Work out the finished part from the listing and answer in its coordinate system (mm). A direction names the side the tool comes from. Give positions to 0.01 mm unless a question says otherwise; leave off trailing zeros. Order: outer loops, then holes, each group sorted by start corner. A loop starts at its lowest first (then second) coordinate and runs counter-clockwise, first axis right, second up.
```python
from build123d import *

# Parameters (mm, degrees)
F0_W        = 65
F0_H        = 56
F1_DEPTH    = 41
F2_T        = -3
F3_W        = 5.12
F3_H        = 12.5
F4_DEPTH    = 4.318
F5_W        = 3.9
F5_H        = 31
F6_DEPTH    = 2
F7_W        = 3.9
F7_H        = 31
F8_DEPTH    = 2
F9_T1_DEPTH = 47.7630546142
F11_DEPTH   = 66.294
F12_W       = 8
F12_H       = 50
F13_DEPTH   = 14.732
F14_W       = 8.89
F14_H       = 2.41
F14_W_2     = 7.2
F15_DEPTH   = 25
F16_W       = 7.2
F16_H       = 2.41
F17_DEPTH   = 0.8
F18_W       = 32.2036024
F18_H       = 3
F19_DEPTH   = 25
F20_W       = 32.2036024
F20_H       = 3
F21_DEPTH   = 3.5
F22_W       = 65
F22_H       = 1.6
F23_DEPTH   = 1
F23_TAPER   = -30
F25_DEPTH   = 0.8
F26_W       = 8.89
F26_H       = 2.41
F27_DEPTH   = 0.8
F28_W       = 0.5773502692
F28_H       = 2.7547005384
F29_DEPTH   = 25
F30_W       = 3
F30_H       = 27.2
F30_H_2     = 28.8
F31_DEPTH   = 6


# Not quite as in the source:
# - a fillet or chamfer that OpenCascade refuses, or shapes differently, is made with other operations: its cross-section is extruded or revolved along the edge and cut away or added


with BuildPart() as f1:
    # F0 (on Top) → F1 (new body)
    with BuildSketch(Plane.XY):
        with Locations((-1.2741552845, -5.3390697837)):
            Rectangle(F0_W, F0_H)
    extrude(amount=F1_DEPTH)

    # F2
    f2_openings = [f1.faces().sort_by_distance(p)[0] for p in [
        (31.225845, -5.33907, 20.5),
    ]]
    offset(amount=F2_T, openings=f2_openings)

    # F3 (on face) → F4 (cut)
    with BuildSketch(Plane(origin=(-33.7741552845, 0, 0), x_dir=(0, -1, 0), z_dir=(-1, 0, 0))):
        with Locations((-7.7209302163, 19.25)):
            Rectangle(F3_W, F3_H)
        with Locations((11.3990697837, 19.25)):
            Rectangle(F3_W, F3_H)
    extrude(amount=-F4_DEPTH, mode=Mode.SUBTRACT)

    # F5 (on face) → F6 (join)
    with BuildSketch(Plane(origin=(0, 22.6609302163, 0), x_dir=(-1, 0, 0), z_dir=(0, 1, 0))):
        with Locations((-24.2758447155, 20.5)):
            Rectangle(F5_W, F5_H)
    extrude(amount=F6_DEPTH)

    # F7 (on face) → F8 (join)
    with BuildSketch(Plane.XZ.offset(33.3390697837)):
        with Locations((24.2758447155, 20.5)):
            Rectangle(F7_W, F7_H)
    extrude(amount=F8_DEPTH)

    # F9: fillet of radius 3.81 on 2 edges, made by hand

    # F9_s2 → F9_t1 (cut)
    with BuildSketch(Plane.XY.offset(-3.3815273071)):
        with BuildLine():
            ThreePointArc((22.3258447155, 22.6609302163), (23.7265335088, 24.1229479424), (25.6784556384, 24.6609302163))
            Line((25.6784556384, 24.6609302163), (22.3258447155, 24.6609302163))
            Line((22.3258447155, 24.6609302163), (22.3258447155, 22.6609302163))
        make_face()
        with BuildLine():
            ThreePointArc((22.3258447155, -33.3390697837), (23.7265335088, -34.8010875098), (25.6784556384, -35.3390697837))
            Line((25.6784556384, -35.3390697837), (22.3258447155, -35.3390697837))
            Line((22.3258447155, -35.3390697837), (22.3258447155, -33.3390697837))
        make_face()
    extrude(amount=F9_T1_DEPTH, mode=Mode.SUBTRACT)

    # F10 (on face) → F11 (cut)
    with BuildSketch(Plane(origin=(0, 22.6609302163, 0), x_dir=(-1, 0, 0), z_dir=(0, 1, 0))):
        Polygon((0.9777576845, 38), (-31.2258447155, 38), (-31.2258447155, 3), (0.9777576845, 3), (0.9777576845, 4), (-28.0222423155, 4), (-28.0222423155, 37), (0.9777576845, 37), align=None)
    extrude(amount=-F11_DEPTH, mode=Mode.SUBTRACT)

    # F12 (on face) → F13 (cut)
    with BuildSketch(Plane.XY.offset(41)):
        with Locations((27.2258447155, -5.3390697837)):
            Rectangle(F12_W, F12_H)
    extrude(amount=-F13_DEPTH, mode=Mode.SUBTRACT)

    # F14 (on face) → F15 (cut)
    with BuildSketch(Plane.XY.offset(41)):
        with Locations((-1.8741552845, 1.0109302163)):
            Rectangle(F14_W, F14_H)
        with BuildLine():
            ThreePointArc((-13.7741552845, -8.0290697837), (-11.8720380431, -7.2411870251), (-11.0841552845, -5.3390697837))
            ThreePointArc((-11.0841552845, -5.3390697837), (-11.8720380431, -3.4369525423), (-13.7741552845, -2.6490697837))
            ThreePointArc((-13.7741552845, -2.6490697837), (-15.6762725259, -3.4369525423), (-16.4641552845, -5.3390697837))
            ThreePointArc((-16.4641552845, -5.3390697837), (-15.6762725259, -7.2411870251), (-13.7741552845, -8.0290697837))
        make_face()
        with Locations((-1.8741552845, -11.6890697837)):
            Rectangle(F14_W_2, F14_H)
        with BuildLine():
            ThreePointArc((-16.4641552845, -5.3390697837), (-15.6762725259, -3.4369525423), (-13.7741552845, -2.6490697837))
            Line((-13.7741552845, -2.6490697837), (-16.4641552845, -2.6490697837))
            Line((-16.4641552845, -2.6490697837), (-16.4641552845, -5.3390697837))
        make_face()
        with BuildLine():
            Line((-16.4641552845, -8.0290697837), (-13.7741552845, -8.0290697837))
            ThreePointArc((-13.7741552845, -8.0290697837), (-15.6762725259, -7.2411870251), (-16.4641552845, -5.3390697837))
            Line((-16.4641552845, -5.3390697837), (-16.4641552845, -8.0290697837))
        make_face()
    extrude(amount=-F15_DEPTH, mode=Mode.SUBTRACT)

    # F16 (on face) → F17 (cut)
    with BuildSketch(Plane(origin=(0, 0, 38), x_dir=(1, 0, 0), z_dir=(0, 0, -1))):
        Polygon((-30.7741552845, 12.0888292812), (-30.7741552845, 11.2888292812), (-8.9876995774, 11.2888292812), (-5.4741552845, 10.0590887787), (1.7258447155, 10.0590887787), (5.2393890084, 11.2888292812), (23.2258447155, 11.2888292812), (23.2258447155, 12.0888292812), (5.2393890084, 12.0888292812), (1.7258447155, 13.3185697837), (-5.4741552845, 13.3185697837), (-8.9876995774, 12.0888292812), align=None)
        with Locations((-1.8741552845, 11.6890697837)):
            Rectangle(F16_W, F16_H, mode=Mode.SUBTRACT)
    extrude(amount=-F17_DEPTH, mode=Mode.SUBTRACT)

    # F18 (on face) → F19 (cut)
    with BuildSketch(Plane(origin=(0, 0, 38), x_dir=(1, 0, 0), z_dir=(0, 0, -1))):
        with Locations((15.1240435155, -21.1609302163)):
            Rectangle(F18_W, F18_H)
        Polygon((-0.9777576845, 33.3390697837), (-0.9777576845, 30.3390697837), (23.2258447155, 30.3390697837), (31.2258447155, 30.3390697837), (31.2258447155, 33.3390697837), align=None)
    extrude(amount=-F19_DEPTH, mode=Mode.SUBTRACT)

    # F20 (on face) → F21 (cut)
    with BuildSketch(Plane(origin=(0, 0, 0), x_dir=(1, 0, 0), z_dir=(0, 0, -1))):
        with Locations((15.1240435155, -21.1609302163)):
            Rectangle(F20_W, F20_H)
        with Locations((15.1240435155, 31.8390697837)):
            Rectangle(F20_W, F20_H)
    extrude(amount=-F21_DEPTH, mode=Mode.SUBTRACT)

    # F22 (on face) → F23 (join)
    with BuildSketch(Plane(origin=(0, 0, 0), x_dir=(1, 0, 0), z_dir=(0, 0, -1))):
        with Locations((-1.2741552845, 5.3390697837)):
            Rectangle(F22_W, F22_H)
    extrude(amount=F23_DEPTH, taper=F23_TAPER)

    # F24 (on face) → F25 (cut)
    with BuildSketch(Plane(origin=(0, 0, 38), x_dir=(1, 0, 0), z_dir=(0, 0, -1))):
        Polygon((23.2258447155, 3.6890697837), (23.2258447155, 6.9890697837), (-8.1741552845, 6.9890697837), (-8.9247106344, 8.2890697837), (-8.9247106344, 8.7890697837), (-19.4271999345, 8.7890697837), (-19.4271999345, 1.8890697837), (-8.9247106344, 1.8890697837), (-8.9247106344, 2.3890697837), (-8.1741552845, 3.6890697837), align=None)
        with BuildLine():
            Line((-16.4641552845, 8.0290697837), (-13.7741552845, 8.0290697837))
            ThreePointArc((-13.7741552845, 8.0290697837), (-11.0841552845, 5.3390697837), (-13.7741552845, 2.6490697837))
            Line((-13.7741552845, 2.6490697837), (-16.4641552845, 2.6490697837))
            Line((-16.4641552845, 2.6490697837), (-16.4641552845, 8.0290697837))
        make_face(mode=Mode.SUBTRACT)
    extrude(amount=-F25_DEPTH, mode=Mode.SUBTRACT)

    # F26 (on face) → F27 (cut)
    with BuildSketch(Plane(origin=(0, 0, 38), x_dir=(1, 0, 0), z_dir=(0, 0, -1))):
        Polygon((-30.7741552845, -0.6106897138), (-30.7741552845, -1.4106897138), (-9.8326995774, -1.4106897138), (-6.3191552845, -2.6404302163), (2.5708447155, -2.6404302163), (6.0843890084, -1.4106897138), (23.2258447155, -1.4106897138), (23.2258447155, -0.6106897138), (6.0843890084, -0.6106897138), (2.5708447155, 0.6190507887), (-6.3191552845, 0.6190507887), (-9.8326995774, -0.6106897138), align=None)
        with Locations((-1.8741552845, -1.0109302163)):
            Rectangle(F26_W, F26_H, mode=Mode.SUBTRACT)
    extrude(amount=-F27_DEPTH, mode=Mode.SUBTRACT)

    # F28 (on face) → F29 (cut)
    with BuildSketch(Plane(origin=(0, 0, -1), x_dir=(1, 0, 0), z_dir=(0, 0, -1))):
        with Locations((-34.0628304191, 5.3390697837)):
            Rectangle(F28_W, F28_H)
    extrude(amount=-F29_DEPTH, mode=Mode.SUBTRACT)

    # F30 (on face) → F31 (join)
    with BuildSketch(Plane(origin=(0, 0, 0), x_dir=(1, 0, 0), z_dir=(0, 0, -1))):
        with Locations((-32.2741552845, 19.7390697837)):
            Rectangle(F30_W, F30_H)
        with Locations((-32.2741552845, -8.2609302163)):
            Rectangle(F30_W, F30_H_2)
    extrude(amount=F31_DEPTH)


solid = f1.part
```
1. Straight lines are drawn through the part: probe 1 along Z at (x, y) = (-19.5, 12.5); probe 2 along Y at (x, z) = (-2.5, 7); probe 3 along X at (y, z) = (-28.5, 35). For each, find the intervals that lie inside material, in ascending order.
Findings below:
probe 1: z = 0 to 3, 38 to 41
probe 2: y = -33.34 to -30.34, 19.66 to 22.66
probe 3: x = -33.77 to -30.77
2. Given P1, Ø4, axis at y = 9.5, z = 9, coming from the +X side; P2, Ø3.5, axis at y = 6.5, z = 1, coming from the +X side; P3, Ø1, axis at y = -34, z = 16.5, coming from the +X side, each flat-ended and moving along its own axis, determine where each tip first touches the part or whether it passes through.
Findings below:
P1: stops at x = -30.77
P2: stops at x = 31.23
P3: stops at x = 26.23
3. The part is cut by section C-C (x = 15.5). State how many separate pieces and enclosed holes the cut face has, then the cut area to 3 significant figures.
Findings below:
separate pieces: 4
enclosed holes: 0
area: 496 mm2
4. Which of the six approach directions +Z, -Z, +X, -X, +Y, -Y give full straight-line access (tool end or side, diameter ignored) to faces 5 (the face through (26.226, -34, 20)), 6 (the face through (-32, 8, 13)), 7 (the face through (-0.978, -32, 39))?
Findings below:
face 5: +Z, -Z, +X, -Y
face 6: +X, -X
face 7: +Z, +X, -Y
5. The part is cut by section B-B (y = 20.5). Write down the section's boundary in (x, z).
Findings below:
outline: (-33.77, -6) - (-30.77, -6) - (-30.77, 0) - (-0.98, 0) - (-0.98, 4) - (28.02, 4) - (28.02, 37) - (-0.98, 37) - (-0.98, 41) - (-33.77, 41) - close
6. The part is cut by section D-D (z = 10). Write down the section's boundary in (x, y), then the cut area to 3 significant figures.
Findings below:
outline: (-33.77, -33.34) - (22.33, -33.34) arc R3.81 ccw to (25.68, -35.34) - (26.23, -35.34) - (26.23, -33.34) - (28.02, -33.34) - (28.02, -30.34) - (-30.77, -30.34) - (-30.77, 19.66) - (28.02, 19.66) - (28.02, 22.66) - (26.23, 22.66) - (26.23, 24.66) - (25.68, 24.66) arc R3.81 ccw to (22.33, 22.66) - (-33.77, 22.66) - close
area: 533 mm2
7. The mould has two halves that part along Z. Classify faces 1 (the face through (-4, 11, 38)), 2 (the face through (23.226, -6, 40)), 3 (the face through (-4, -21, 38)), 4 (the face through (14, -32, 37)): pulls with the +Z half, pulls with the -Z half, needs draft (parallel to the pull), parting line crosses it, or undercut.
Findings below:
face 1: undercut
face 2: needs draft
face 3: undercut
face 4: pulls with the +Z half
8. The part is cut by section A-A (z = 21). Write down the section's boundary in (x, y), then the cut area to 3 significant figures.
Findings below:
outline: (-33.77, -33.34) - (22.33, -33.34) arc R3.81 ccw to (25.68, -35.34) - (26.23, -35.34) - (26.23, -33.34) - (28.02, -33.34) - (28.02, -30.34) - (-30.77, -30.34) - (-30.77, -13.96) - (-33.77, -13.96) - close; (-33.77, -8.84) - (-30.77, -8.84) - (-30.77, 5.16) - (-33.77, 5.16) - close; (-33.77, 10.28) - (-30.77, 10.28) - (-30.77, 19.66) - (28.02, 19.66) - (28.02, 22.66) - (26.23, 22.66) - (26.23, 24.66) - (25.68, 24.66) arc R3.81 ccw to (22.33, 22.66) - (-33.77, 22.66) - close
area: 502 mm2
